Read the model definition and answer for the solid it produces. Units are mm, in the model's axes. Face numbers are marked on the shaded views. Give positions to 0.01 mm unless a question says otherwise; leave off trailing zeros. Order: outer loops, then holes, each group sorted by start corner. A loop starts at its lowest first (then second) coordinate and runs counter-clockwise, first axis right, second up. Notation, with made-up numbers: M -19,15 L 16,15 A34 cw 16,53 Z; hole C 58.5,46.25 d4. An arc over 180 degrees is marked long. One line per item, written item: value.
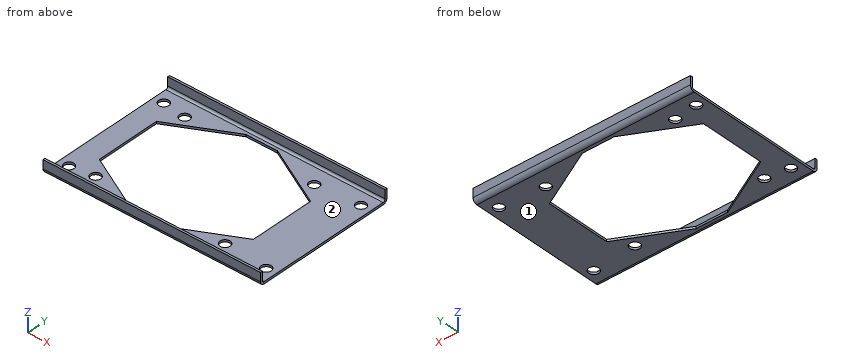
from build123d import *

# Parameters (mm, degrees)
SM_BASE_FLANGE_1_DEPTH           = 3
SM_EDGE_FLANGE_1_STRIP_W         = 18
SM_EDGE_FLANGE_1_STRIP_H         = 3
SM_EDGE_FLANGE_1_STRIP_CUT_DEPTH = 302
SM_EDGE_FLANGE_1_DEPTH           = 302
SKETCH_9_R                       = 7
CUT_EXTRUDE_1_DEPTH              = 10
SKETCH_10_R                      = 7
CUT_EXTRUDE_2_DEPTH              = 3


# Sheet-metal steps are written as plain solids
with BuildPart() as part:
    # Sketch 1 → Базовая кромка1 (new body)
    with BuildSketch(Plane.XY):
        Polygon((-151, 0), (151, 0), (151, 96.5), (93, 96.5), (93, 51.5), (8, 7.25), (-36, 7.25), (-121, 51.5), (-121, 96.5), (-151, 96.5), align=None)
    extrude(amount=-SM_BASE_FLANGE_1_DEPTH)

    # Ребро-кромка1 strip (across the edge) → Ребро-кромка1 strip cut (cut)
    with BuildSketch(Plane.YZ.offset(-151)):
        with Locations((-6, -1.5)):
            Rectangle(SM_EDGE_FLANGE_1_STRIP_W, SM_EDGE_FLANGE_1_STRIP_H)
    extrude(amount=SM_EDGE_FLANGE_1_STRIP_CUT_DEPTH, mode=Mode.SUBTRACT)

    # Ребро-кромка1 section (across the edge) → Ребро-кромка1 (add)
    with BuildSketch(Plane.YZ.offset(-151)):
        with BuildLine():
            Line((-3, 3), (-3, 15))
            Line((-3, 15), (0, 15))
            Line((0, 15), (0, 3))
            ThreePointArc((0, 3), (0.878679656, 0.878679656), (3, 0))
            Line((3, 0), (3, -3))
            ThreePointArc((3, -3), (-1.242640687, -1.242640687), (-3, 3))
        make_face()
    extrude(amount=SM_EDGE_FLANGE_1_DEPTH)

    # Зеркальное отражение1: part across plane


with BuildPart() as part_1:
    add(part.part)
    add(part.part.mirror(Plane(origin=(-151, 96.5, -3), x_dir=(0, 0, 1), z_dir=(0, 1, 0))))

    # Эскиз9 → Вырез-Вытянуть1 (cut)
    with BuildSketch(Plane(origin=(0, 0, -3), x_dir=(-1, 0, 0), z_dir=(0, 0, -1))):
        with Locations((137, 171)):
            Circle(SKETCH_9_R)
        with Locations((137, 22)):
            Circle(SKETCH_9_R)
        with Locations(Location((-137, 22, 0), (0, 0, 180))):
            Circle(SKETCH_9_R)
        with Locations(Location((-137, 171, 0), (0, 0, 180))):
            Circle(SKETCH_9_R)
    extrude(amount=-CUT_EXTRUDE_1_DEPTH, mode=Mode.SUBTRACT)

    # Эскиз10 → Вырез-Вытянуть2 (cut)
    with BuildSketch(Plane.XY):
        with Locations((76, 166.5)):
            Circle(SKETCH_10_R)
        with Locations((-104, 166.5)):
            Circle(SKETCH_10_R)
        with Locations((-104, 26.5)):
            Circle(SKETCH_10_R)
        with Locations((76, 26.5)):
            Circle(SKETCH_10_R)
    extrude(amount=-CUT_EXTRUDE_2_DEPTH, mode=Mode.SUBTRACT)


solid = part_1.part
1) Find section D-D, the plane z = 8. Write down the section's boundary in (x, y), plus the area to 3 significant figures.
Reported:
outline: M -151,-3 L 151,-3 L 151,0 L -151,0 Z; M -151,193 L 151,193 L 151,196 L -151,196 Z
area: 1,810 mm^2
2) Determine the mould class of the marked faces 1 and 2 for opening direction Y: +Y half, -Y half, draft (parallel to the pull), parting line (faces both ways), or undercut.
Reported:
face 1: draft
face 2: undercut
3) Each of these flat-tipped pins is pushed along its axis until it touches: pin 1 Ø1.5 at (x, z) = (-17, -1) entering from -Y; pin 2 Ø16 at (x, y) = (-104, 166.5) entering from -Z; pin 3 Ø16 at (x, y) = (-104, 26.5) entering from +Z; pin 4 Ø1.5 at (x, z) = (0, 1.5) entering from -Y. Where does it stop, or does it pass through?
Reported:
pin 1: stops at y = -2.04
pin 2: stops at z = -3
pin 3: stops at z = 0
pin 4: stops at y = -2.95
4) Find section B-B, the plane y = 58.5. Write down the section's boundary in (x, z), plus the area to 3 significant figures.
Reported:
outline: M -151,-3 L -121,-3 L -121,0 L -151,0 Z; M 93,-3 L 151,-3 L 151,0 L 93,0 Z
area: 264 mm^2
5) Find section C-C, the plane x = -137. Write down the section's boundary in (y, z), plus the area to 3 significant figures.
Reported:
outline: M -3,3 A6 ccw 3,-3 L 15,-3 L 15,0 L 3,0 A3 cw 0,3 L 0,15 L -3,15 Z; M 29,-3 L 164,-3 L 164,0 L 29,0 Z; M 178,-3 L 190,-3 A6 ccw 196,3 L 196,15 L 193,15 L 193,3 A3 cw 190,0 L 178,0 Z
area: 591 mm^2
6) Consider probe 1 along Y at (x, z) = (127.5, 7.25); probe 2 along Y at (x, z) = (76, -2.3); probe 3 along Y at (x, z) = (76, -0.8). Determine where each line is inside the solid, lowest interval first.
Reported:
probe 1: y = -3 to 0, 193 to 196
probe 2: y = 0.19 to 19.5, 33.5 to 42.65, 150.35 to 159.5, 173.5 to 192.81
probe 3: y = -1.64 to 19.5, 33.5 to 42.65, 150.35 to 159.5, 173.5 to 194.64
7) Find section A-A, the plane x = 76. Write down the section's boundary in (y, z).
Reported:
outline: M -3,3 A6 ccw 3,-3 L 19.5,-3 L 19.5,0 L 3,0 A3 cw 0,3 L 0,15 L -3,15 Z; M 33.5,-3 L 42.65,-3 L 42.65,0 L 33.5,0 Z; M 150.35,-3 L 159.5,-3 L 159.5,0 L 150.35,0 Z; M 173.5,-3 L 190,-3 A6 ccw 196,3 L 196,15 L 193,15 L 193,3 A3 cw 190,0 L 173.5,0 Z
